The model under review builds one solid part; all positions refer to its coordinate system, in mm. A direction names the side the tool comes from. Round coordinates to 2 decimals unless told otherwise and drop trailing zeros. Write each loop counter-clockwise with the first axis right and the second up, starting at its lowest first coordinate (ties: lowest second). Pieces come first, ordered by that corner, then holes. Notation, with made-up numbers: M 58,5.5 L 77,5.5 A23 cw 77,31.5 Z; hole C -27,-18.5 d10. An arc over 180 degrees is marked long. One line per item, written item: value. Start each with the question number.
1) Wall thickness on probe 1 along Y at (x, z) = (14, 0); probe 2 along Z at (x, y) = (21.5, -37); probe 3 along Z at (x, y) = (5, 19): over which ranges is each line inside the solid? List them lowest first.
2) Tool access review of faces 1 (the face through (24.65, 27.702, -24.727)), 2 (the face through (24.65, 36.91, 4.04)), 3 (the face through (24.65, 20.937, 23.198)), 4 (the face through (24.65, -27.568, 25.115)): name each direction out of +Z, -Z, +X, -X, +Y, -Y from which nothing blocks a thin tool from reaching the whole face with its end or side.
3) Take a section at A-A, the plane z = 0. Write out the cut boundary in (x, y).
4) For P1, Ø5, axis at x = 37, z = -23.5, coming from the +Y side; P2, Ø3, axis at x = 9.5, z = -2.5, coming from the -Y side; P3, Ø1.2, axis at x = 20.5, y = 13.5, coming from the +Z side, all flat-tipped, find the tip position at first contact; note any pin that passes through.
5) Take a section at B-B, the plane y = -34.5. Write out the cut boundary in (x, z), and give its area (3 significant figures).
6) Take a section at C-C, the plane y = -19.5. Write out the cut boundary in (x, z), and give its area (3 significant figures).
7) Mouldability with a two-part tool opening along Z and no side actions: class faces 5 (the face through (25.35, -12.99, 0.51)), 6 (the face through (25.35, -13.148, -40.415)), 7 (the face through (25.35, 41.575, 8.821)), 8 (the face through (24.65, -30.56, 6.53)) as +Z half, -Z half, draft (parallel to the pull), parting line (faces both ways), or undercut.
from build123d import *

# Parameters (mm, degrees)
BASPROSKE_W     = 50
BASPROSKE_H     = 42.5
TOOTHCUT_DEPTH  = 79.182478856
TEETHCUTS_COUNT = 15
TEETHCUTS_ANGLE = 336
BORSKE_R        = 13
BORE_DEPTH      = 50.0000508
KEYSKE_W        = 8
KEYSKE_H        = 16.3
KEYWAY_DEPTH    = 50.0000508


with BuildPart() as part:
    # BasProSke → Base-Revolve (revolve)
    with BuildSketch(Plane(origin=(0, 0, 0), x_dir=(1, 0, 0), z_dir=(0, 1, 0)), mode=Mode.PRIVATE) as base_revolve_sk:
        with Locations((25, 21.25)):
            Rectangle(BASPROSKE_W, BASPROSKE_H)
    revolve(base_revolve_sk.sketch.rotate(Axis((-10, 0, 0), (1, 0, 0)), 180), axis=Axis((-10, 0, 0), (1, 0, 0)))

    # TooCutSke → ToothCut (cut, through all)
    with BuildSketch(Plane(origin=(0, 0, 0), x_dir=(0, 0, -1), z_dir=(1, 0, 0))):
        with BuildLine():
            ThreePointArc((2.624472836, 31.138595719), (0, 31.249), (-2.624472836, 31.138595719))
            ThreePointArc((-2.624472836, 31.138595719), (-4.084227986, 37.002862003), (-7.739685892, 41.815151649))
            ThreePointArc((-7.739685892, 41.815151649), (0, 42.5254), (7.739685892, 41.815151649))
            ThreePointArc((7.739685892, 41.815151649), (4.084227986, 37.002862003), (2.624472836, 31.138595719))
        make_face()
    toothcut = extrude(amount=TOOTHCUT_DEPTH, mode=Mode.SUBTRACT)

    # TeethCuts: ToothCut ×15 about axis
    teethcuts_axis = Axis((-10, 0, 0), (1, 0, 0))
    for i in range(1, TEETHCUTS_COUNT):
        add(toothcut.rotate(teethcuts_axis, i * TEETHCUTS_ANGLE / (TEETHCUTS_COUNT - 1)), mode=Mode.SUBTRACT)

    # BorSke → Bore (cut, symmetric)
    with BuildSketch(Plane(origin=(0, 0, 0), x_dir=(0, 0, -1), z_dir=(1, 0, 0))):
        with Locations(Location((0, 0, 0), (0, 0, 180))):
            Circle(BORSKE_R)
    extrude(amount=BORE_DEPTH, both=True, mode=Mode.SUBTRACT)

    # KeySke → Keyway (cut, symmetric)
    with BuildSketch(Plane(origin=(0, 0, 0), x_dir=(0, 0, -1), z_dir=(1, 0, 0))):
        with Locations((0, 8.15)):
            Rectangle(KEYSKE_W, KEYSKE_H)
    extrude(amount=KEYWAY_DEPTH, both=True, mode=Mode.SUBTRACT)


solid = part.part
Checked values:
1. probe 1: y = -42.5 to -13, 16.3 to 31.25
1. probe 2: z = -18.56 to -13.17, -3.71 to 3.71, 13.17 to 18.56
1. probe 3: z = -36.75 to -25.04, -24.81 to 24.81, 25.04 to 36.75
2. face 1: -Z, +X, -X
2. face 2: +X, -X, +Y
2. face 3: +X, -X
2. face 4: +X, -X, -Y
3. outline: M 0,-42.5 L 50,-42.5 L 50,-13 L 0,-13 Z; M 0,16.3 L 50,16.3 L 50,31.25 L 0,31.25 Z
4. P1: stops at y = 35.04
4. P2: stops at y = -42.49
4. P3: stops at z = 32.48
5. outline: M 0,-18.68 L 50,-18.68 L 50,-11.08 L 0,-11.08 Z; M 0,-4.09 L 50,-4.09 L 50,4.09 L 0,4.09 Z; M 0,11.08 L 50,11.08 L 50,18.68 L 0,18.68 Z
5. area: 1,170 mm2
6. outline: M 0,-27.81 L 50,-27.81 L 50,27.81 L 0,27.81 Z
6. area: 2,780 mm2
7. face 5: undercut
7. face 6: -Z half
7. face 7: +Z half
7. face 8: undercut
